from build123d import *

# Parameters (mm, degrees)
BOSS_EXTRUDE1_DEPTH = 23
SKETCH4_R           = 5
CUT_EXTRUDE3_DEPTH  = 28
CUT_EXTRUDE4_DEPTH  = 9


with BuildPart() as part:
    # Sketch1 → Boss-Extrude1 (new body)
    with BuildSketch(Plane.XY):
        with BuildLine():
            Line((-26.278110913, -11.347842937), (-28.372166089, -9.043842083))
            Line((-28.372166089, -9.043842083), (-7.990208081, 9.462215656))
            ThreePointArc((-7.990208081, 9.462215656), (-6.229501786, 11.136017118), (-3.800938061, 11.07456612))
            Line((-3.800938061, 11.07456612), (-3.637536714, 11.001987755))
            Line((-3.637536714, 11.001987755), (19.793985679, 9.88969345))
            ThreePointArc((19.793985679, 9.88969345), (28.356197765, 0.474073738), (18.940578052, -8.088138348))
            Line((18.940578052, -8.088138348), (15.348738563, -7.91649311))
            ThreePointArc((15.348738563, -7.91649311), (14.978028358, -7.825889172), (14.668239185, -7.603030926))
            Line((14.668239185, -7.603030926), (5.35012395, 2.296550983))
            Line((5.35012395, 2.296550983), (-3.419163159, 5.255947346))
            ThreePointArc((-3.419163159, 5.255947346), (-4.191805611, 4.94513719), (-5.014133862, 4.813396687))
            Line((-5.014133862, 4.813396687), (-26.278110913, -11.347842937))
        make_face()
    extrude(amount=BOSS_EXTRUDE1_DEPTH)

    # Sketch4 → Cut-Extrude3 (cut)
    with BuildSketch(Plane(origin=(0, 0, 0), x_dir=(-1, 0, 0), z_dir=(0, 0, -1))):
        with Locations((-19.367281866, 0.900777551)):
            Circle(SKETCH4_R)
    extrude(amount=-CUT_EXTRUDE3_DEPTH, mode=Mode.SUBTRACT)

    # Sketch5 → Cut-Extrude4 (cut)
    with BuildSketch(Plane(origin=(0, 0, 0), x_dir=(-1, 0, 0), z_dir=(0, 0, -1))):
        with BuildLine():
            Line((-8.280771458, 10.715087027), (-20.34194177, 10.142544005))
            ThreePointArc((-20.34194177, 10.142544005), (-28.752978591, 0.302154859), (-18.904257366, -8.099124161))
            Line((-18.904257366, -8.099124161), (-15.316689911, -7.927683074))
            ThreePointArc((-15.316689911, -7.927683074), (-14.945947651, -7.837064321), (-14.636142172, -7.614169396))
            Line((-14.636142172, -7.614169396), (-5.318075302, 2.285361131))
            ThreePointArc((-5.318075302, 2.285361131), (-6.00282629, 6.780194646), (-8.280771458, 10.715087027))
        make_face()
    extrude(amount=-CUT_EXTRUDE4_DEPTH, mode=Mode.SUBTRACT)


solid = part.part
Read the model definition and answer for the solid it produces. Units are mm, in the model's axes. A direction names the side the tool comes from. Coordinates: 2 decimals unless noted, no trailing zeros. Write each loop counter-clockwise with the first axis right and the second up, starting at its lowest first coordinate (ties: lowest second). Pieces come first, ordered by that corner, then holes. Notation, with made-up numbers: (-22, 76.5) -> (25, 76.5) arc R26 cw to (25, 109.5) -> close; hole circle Ø11 at (-5, 20). An arc over 180 degrees is marked (long way). Return JSON: item names as keys, results as strings.
(1) Which of the six approach directions +Z, -Z, +X, -X, +Y, -Y give full straight-line access (tool end or side, diameter ignored) to faces 4 (the flat face through (5.311, 10.577, 13.895)), 5 (the cylindrical face through (-4.18, 4.95, 11.34))?
Answers below:
{"face 4": "+Z, -Z, +X, +Y", "face 5": "+Z, -Z, -Y"}
(2) Each of these flat-tipped pins is pushed along its axis until it touches: P1, Ø6, axis at x = -16.5, z = 9, coming from the -Y side; P2, Ø3, axis at x = 21, y = 7, coming from the -Z side; P3, Ø3, axis at x = 0, z = 17.5, coming from the -Y side. Where does it stop, or does it pass through?
Answers below:
{"P1": "y = -6.2", "P2": "z = 9", "P3": "y = 3.6"}
(3) Consider line 1 along X through (y, z) = (1.75, 13.25); line 2 along Y through (x, z) = (19.5, 11); line 3 along Y through (x, z) = (15, 16). Determine where each line is inside the solid, lowest interval first. Write a range as from..to.
Answers below:
{"line 1": "-16.48..-9.04, 5.86..14.44, 24.29..28.33", "line 2": "-8.1..-4.1, 5.9..9.9", "line 3": "-7.84..-1.53, 3.34..10.12"}
(4) The part is cut by section D-D on y = 3. Give the vertices of the cut face in (x, z).
Answers below:
{"outline": "(-15.11, 0) -> (-7.4, 0) -> (-7.4, 23) -> (-15.11, 23) -> close; (3.27, 0) -> (5.31, 0) -> (5.31, 9) -> (14.83, 9) -> (14.83, 23) -> (3.27, 23) -> close; (23.91, 9) -> (28.12, 9) -> (28.12, 23) -> (23.91, 23) -> close"}
(5) The part is cut by section C-C on z = 2.25. Give the vertices of the cut face in (x, y).
Answers below:
{"outline": "(-28.37, -9.04) -> (-26.28, -11.35) -> (-5.01, 4.81) arc R3.73 ccw to (-3.42, 5.26) -> (5.32, 2.31) arc R12.24 cw to (8.06, 10.45) -> (-3.64, 11) -> (-3.8, 11.07) arc R3.17 ccw to (-7.99, 9.46) -> close"}
(6) The part is cut by section A-A on y = -1. Give the vertices of the cut face in (x, z), then the cut area to 3 significant figures.
Answers below:
{"outline": "(-19.51, 0) -> (-12.66, 0) -> (-12.66, 23) -> (-19.51, 23) -> close; (8.45, 9) -> (14.74, 9) -> (14.74, 23) -> (8.45, 23) -> close; (23.99, 9) -> (28.16, 9) -> (28.16, 23) -> (23.99, 23) -> close", "area": "304 mm^2"}
(7) The part is cut by section B-B on z = 10.75. Give the vertices of the cut face in (x, y), then the cut area to 3 significant figures.
Answers below:
{"outline": "(-28.37, -9.04) -> (-26.28, -11.35) -> (-5.01, 4.81) arc R3.73 ccw to (-3.42, 5.26) -> (5.35, 2.3) -> (14.67, -7.6) arc R1 ccw to (15.35, -7.92) -> (18.94, -8.09) arc R9 ccw to (19.79, 9.89) -> (-3.64, 11) -> (-3.8, 11.07) arc R3.17 ccw to (-7.99, 9.46) -> close; hole circle Ø10 at (19.37, 0.9)", "area": "453 mm^2"}
(8) For a pull along X with two mould halves and no side action, classify faces 1 (the flat face through (10.07, -2.72, 15.9)), 2 (the flat face through (-18.3, 0.1, 11.3)), 3 (the flat face through (-9, 3, 0)) as pulls with the +X half, pulls with the -X half, needs draft (parallel to the pull), parting line crosses it, or undercut.
Answers below:
{"face 1": "undercut", "face 2": "pulls with the -X half", "face 3": "needs draft"}
